from build123d import *

# Parameters (mm, degrees)
EXTRUDE_1_DEPTH = 10
CHAMFER_1_SIZE  = 2


with BuildPart() as part:
    # 草图1 → 凸台-拉伸1 (new body)
    with BuildSketch(Plane(origin=(0, 0, 0), x_dir=(1, 0, 0), z_dir=(0, 1, 0))):
        with BuildLine():
            Line((0, 6), (20, 6))
            ThreePointArc((20, 6), (26, 0), (20, -6))
            Line((20, -6), (0, -6))
            ThreePointArc((0, -6), (-6, 0), (0, 6))
        make_face()
    extrude(amount=EXTRUDE_1_DEPTH)

    # 草图2 → 切除-旋转1 (revolve, cut)
    with BuildSketch(Plane.XY):
        Polygon((0, 10), (-2.55, 10), (-2.55, 5), (-1.6, 5), (-1.6, 2), (-2.55, 2), (-2.55, 0), (0, 0), align=None)
    revolve(axis=Axis((0, 0, 0), (0, 1, 0)), mode=Mode.SUBTRACT)

    # 草图4 → 切除-旋转2 (revolve, cut)
    with BuildSketch(Plane.XY):
        Polygon((20, 10), (17, 10), (17, 5), (17.425, 5), (17.425, 0), (20, 0), align=None)
    revolve(axis=Axis((20, 0, 0), (0, 1, 0)), mode=Mode.SUBTRACT)

    # 倒角1
    chamfer_1_edges = [part.edges().sort_by_distance(p)[0] for p in [
        (26, 10, 0),
        (10, 10, -6),
        (-6, 10, 0),
        (10, 10, 6),
    ]]
    chamfer(chamfer_1_edges, length=CHAMFER_1_SIZE)


solid = part.part
Input: part model. Units: mm. Frame: model coordinates. A direction names the side the tool comes from. Coordinates: 2 decimals unless noted, no trailing zeros. Loops run counter-clockwise (first coordinate to the right, second up) from the corner with the lowest first, then second, coordinate; pieces in that order, holes last. Notation, with made-up numbers: (69.25, 70) -> (97.25, 70) arc R25 cw to (97.25, 93) -> close; hole circle Ø7 at (-4, 32.5). An arc over 180 degrees is marked (long way). Write each question's results on one line, items separated by ' | '. Start each with the question number.
Q1. Section A-A, the plane z = 0. Return the cut outline in (x, y) (3 decimals).
Q2. Section C-C, the plane x = 3. Return the cut outline in (y, z), plus the area to 3 significant figures.
Q3. Pin query (flat end, axial travel): pin 1 (4.5 mm diameter, centred on x = 0, z = 0, fed in from -Y); pin 2 (1.5 mm diameter, centred on x = 1, z = -1, fed in from +Y); pin 3 (1.5 mm diameter, centred on y = 1.5, z = -4.5, fed in from +X); pin 4 (5 mm diameter, centred on x = 20, z = 0, fed in from -Y). Return the tip coordinate at first contact, or that it passes through.
Q4. Ray query, line 1 (Z direction, x = 20, y = 2.25) (3 decimals); line 2 (X direction, y = 5.5, z = -1.25); line 3 (X direction, y = 3, z = 0.5). Return the intervals inside material, ascending. Write a range as from..to.
Q5. Reachability of faces 4 (the flat face through (2, 2, 0)), 5 (the flat face through (10, 10, 0)), 6 (the cylindrical face through (-1.18, 7.46, -2.26)) from +Z, -Z, +X, -X, +Y, -Y: full face, straight path, thin tool, end or side. Return the list, or none.
Q6. Section B-B, the plane y = 6. Return the cut outline in (x, z), plus the area to 3 significant figures.
Q7. Section D-D, the plane y = 4.5. Return the cut outline in (x, z) (3 decimals), plus the area to 3 significant figures.
Q8. Pull-direction query (Z, two-part tool) for faces 1 (the flat face through (10, 0, 0)), 2 (the cylindrical face through (17.544, 2.465, 0.773)), 3 (the cylindrical face through (26, 4, 0)); classes: released by +Z, released by -Z, zero draft, split by the parting line, or undercut.
Found:
1) outline: (-6, 0) -> (-2.55, 0) -> (-2.55, 2) -> (-1.6, 2) -> (-1.6, 5) -> (-2.55, 5) -> (-2.55, 10) -> (-4, 10) -> (-6, 8) -> close; (1.6, 2) -> (2.55, 2) -> (2.55, 0) -> (17.425, 0) -> (17.425, 5) -> (17, 5) -> (17, 10) -> (2.55, 10) -> (2.55, 5) -> (1.6, 5) -> close; (22.575, 0) -> (26, 0) -> (26, 8) -> (24, 10) -> (23, 10) -> (23, 5) -> (22.575, 5) -> close
2) outline: (0, -6) -> (8, -6) -> (10, -4) -> (10, 4) -> (8, 6) -> (0, 6) -> close | area: 116 mm2
3) pin 1: y = 2 | pin 2: y = 5 | pin 3: x = 24.68 | pin 4: through
4) line 1: -6..-2.575, 2.575..6 | line 2: -5.87..-2.22, 2.22..17.27, 22.73..25.87 | line 3: -5.98..-1.52, 1.52..17.47, 22.53..25.98
5) face 4: -Y | face 5: +Z, -Z, +X, -X, +Y | face 6: +Y
6) outline: (0, -6) -> (20, -6) arc R6 ccw to (20, 6) -> (0, 6) arc R6 ccw to start; hole circle Ø5.1 at (0, 0); hole circle Ø6 at (20, 0) | area: 304 mm2
7) outline: (0, -6) -> (20, -6) arc R6 ccw to (20, 6) -> (0, 6) arc R6 ccw to start; hole circle Ø3.2 at (0, 0); hole circle Ø5.15 at (20, 0) | area: 324 mm2
8) face 1: zero draft | face 2: undercut | face 3: split by the parting line
